Check sheet for the drawn part. Datum: minimum x, y, z corner. Units: mm. A direction names the side the tool comes from. Coordinates: 2 decimals unless noted, no trailing zeros. Loops run counter-clockwise (first coordinate to the right, second up) from the corner with the lowest first, then second, coordinate; pieces in that order, holes last.
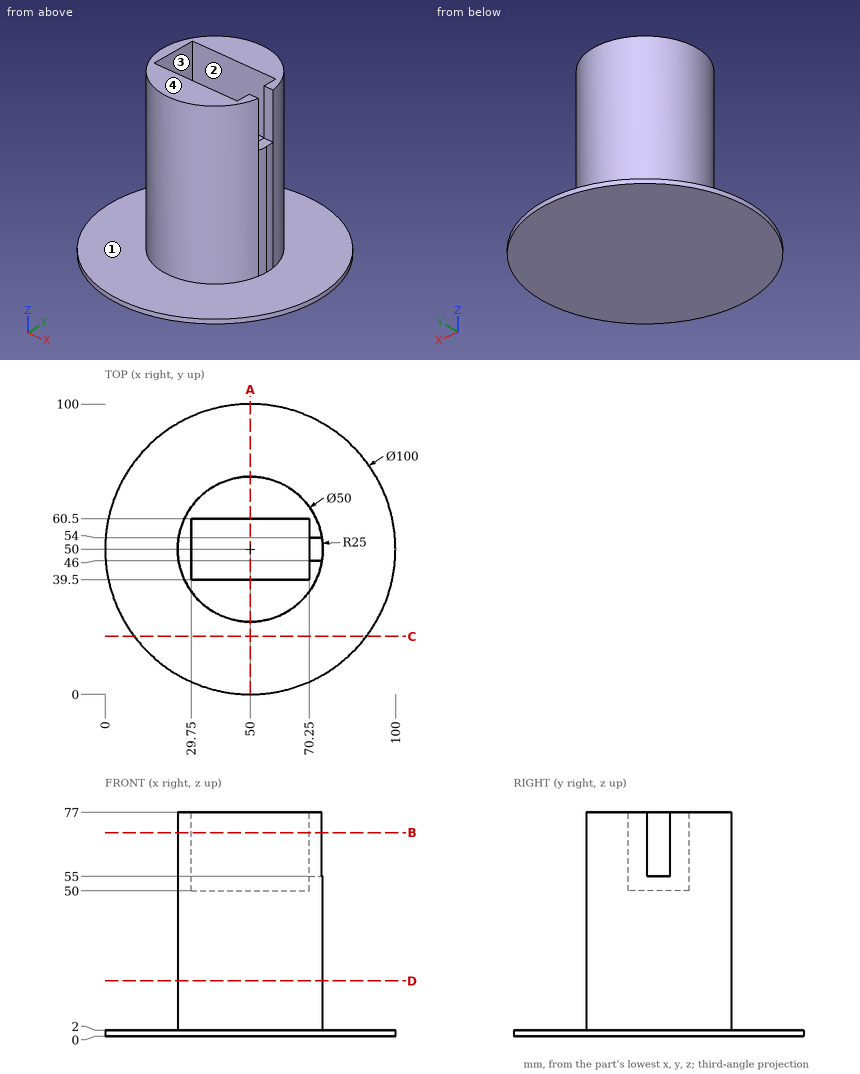
(1) Access from +Z, -Z, +X, -X, +Y, -Y to the whole of each face (thin tool, end or side, straight path). Record for the marked faces 3 and 4.
Findings:
face 3: +Z
face 4: +Z, +X, -X, +Y, -Y
(2) Draft check along Y on the marked faces 1 and 2. Enter one of: +Y half, -Y half, draft (parallel to the pull), parting line (faces both ways), or undercut.
Findings:
face 1: draft
face 2: undercut
(3) Sectioned sample at B-B on z = 70. Record the cut outline in (x, y).
Findings:
outline: (29.75, 39.5) - (29.75, 60.5) - (70.25, 60.5) - (70.25, 54) - (74.68, 54) arc R25 ccw (long way) to (74.68, 46) - (70.25, 46) - (70.25, 39.5) - close
(4) Gauge pin test, flat ends, axial feed: pin 1 Ø2 at (y, z) = (29.5, 32) entering from +X; pin 2 Ø1.3 at (x, z) = (72, 68) entering from +Y; pin 3 Ø1 at (x, y) = (24.5, 60) entering from +Z. Record the tip position at first contact, or that the pin passes through.
Findings:
pin 1: stops at x = 65.64
pin 2: stops at y = 63.01
pin 3: stops at z = 2
(5) Scan lines: L1, parallel to Z at x = 75, y = 21; L2, parallel to Z at x = 60, y = 50; L3, parallel to X at y = 49, z = 18. Record each from-to range of solid material in increasing order.
Findings:
L1: z = 0 to 2
L2: z = 0 to 50
L3: x = 25.02 to 74.98
(6) Sectioned sample at D-D on z = 19. Record the cut outline in (x, y).
Findings:
outline: circle Ø50 at (50, 50)
(7) Sectioned sample at A-A on x = 50. Record the cut outline in (y, z), and give its area (3 significant figures).
Findings:
outline: (0, 0) - (100, 0) - (100, 2) - (75, 2) - (75, 77) - (60.5, 77) - (60.5, 50) - (39.5, 50) - (39.5, 77) - (25, 77) - (25, 2) - (0, 2) - close
area: 3,380 mm2
(8) Sectioned sample at C-C on y = 20. Record the cut outline in (x, z), and give its area (3 significant figures).
Findings:
outline: (10, 0) - (90, 0) - (90, 2) - (10, 2) - close
area: 160 mm2
